```python
from build123d import *

# Parameters (mm, degrees)
TOP_BOW_EXTRUSION_DEPTH              = 56.86004
PORT_STARBOARD_CUT_DEPTH             = 38.529378828
PORT_STARBOARD_CUT_DEPTH_BACK        = 38.529527124
FORE_AFT_BOW_WRAPUP_EXTRUSTION_REACH = 76.36
SCALE_2_SCALE                        = 2
SHELL2_T                             = 2.54


with BuildPart() as part:
    # Cross-Section C Sketch → Fore-Aft Loft section 0
    with BuildSketch(Plane.XY.offset(76.2)):
        Polygon((-0.000593186, -30.406404979), (37.528192355, -12.906444879), (37.528192355, 26.453635249), (-37.529378728, 26.453635249), (-37.529378728, -12.906444879), align=None)
    # Cross-Section B Sketch → Fore-Aft Loft section 1
    with BuildSketch(Plane.XY):
        Polygon((-0.000593186, -30.406404979), (37.528192355, -12.906444879), (37.528192355, 26.453635249), (-37.529378728, 26.453635249), (-37.529378728, -12.906444879), align=None)
    # Cross-Section A Sketch → Fore-Aft Loft section 2
    with BuildSketch(Plane(origin=(0, 0, -76.2), x_dir=(-1, 0, 0), z_dir=(0, 0, -1))):
        Polygon((-0.000593186, -30.406404979), (37.528192355, -12.906444879), (37.528192355, 26.453635249), (-37.529378728, 26.453635249), (-37.529378728, -12.906444879), align=None)
    loft()

    # Top Bow Profile → Top Bow Extrusion (add)
    with BuildSketch(Plane(origin=(0, 26.453635249, 0), x_dir=(1, 0, 0), z_dir=(0, 1, 0))):
        Polygon((37.529378728, 76.2), (0, 150.560276873), (-37.528192355, 76.2), align=None)
    extrude(amount=-TOP_BOW_EXTRUSION_DEPTH)

    # Port-Starboard Profile → Port-Starboard Cut (cut, two sides)
    with BuildSketch(Plane(origin=(0, 0, 0), x_dir=(0, 0, -1), z_dir=(1, 0, 0))) as port_starboard_cut_sk:
        with BuildLine():
            ThreePointArc((76.2, -30.406404979), (122.925878209, -14.460087823), (150.560276873, 26.453635249))
            Line((150.560276873, 26.453635249), (150.560276873, -30.406404979))
            Line((150.560276873, -30.406404979), (76.2, -30.406404979))
        make_face()
    extrude(amount=PORT_STARBOARD_CUT_DEPTH, mode=Mode.SUBTRACT)
    extrude(port_starboard_cut_sk.sketch, amount=-PORT_STARBOARD_CUT_DEPTH_BACK, mode=Mode.SUBTRACT)

    # Fore-Aft Bow Construction Sketch → Fore-aft bow wrapup extrustion (cut, up to next)
    with BuildSketch(Plane.XY.offset(-76.2), mode=Mode.PRIVATE) as fore_aft_bow_wrapup_extrustion_sk1:
        Polygon((0.000593186, -30.406404979), (37.529378728, -30.406404979), (37.529378728, -12.906444879), align=None)
    fore_aft_bow_wrapup_extrustion_tool1 = extrude(fore_aft_bow_wrapup_extrustion_sk1.sketch, amount=-FORE_AFT_BOW_WRAPUP_EXTRUSTION_REACH, mode=Mode.PRIVATE) & part.part
    add(fore_aft_bow_wrapup_extrustion_tool1.solids().sort_by_distance((25.019784, -24.573085, -76.2))[0], mode=Mode.SUBTRACT)
    # Fore-Aft Bow Construction Sketch → Fore-aft bow wrapup extrustion (cut, up to next)
    with BuildSketch(Plane.XY.offset(-76.2), mode=Mode.PRIVATE) as fore_aft_bow_wrapup_extrustion_sk2:
        Polygon((-37.528192355, -30.406404979), (0.000593186, -30.406404979), (-37.528192355, -12.906444879), align=None)
    fore_aft_bow_wrapup_extrustion_tool2 = extrude(fore_aft_bow_wrapup_extrustion_sk2.sketch, amount=-FORE_AFT_BOW_WRAPUP_EXTRUSTION_REACH, mode=Mode.PRIVATE) & part.part
    add(fore_aft_bow_wrapup_extrustion_tool2.solids().sort_by_distance((-25.018597, -24.573085, -76.2))[0], mode=Mode.SUBTRACT)


with BuildPart() as part_1:
    # Scale 2: scaled about (-0.000240035, 2.235376986, -18.845056047)
    add(part.part.scale(SCALE_2_SCALE).moved(Location((0.000240035, -2.235376986, 18.845056047))))

    # Shell2 (no face opened: a closed hollow body)
    add(offset(amount=-SHELL2_T, mode=Mode.PRIVATE), mode=Mode.SUBTRACT)


solid = part_1.part
```
Source: CAD feature listing. Evaluate the final solid. Frame: model axes, mm. A direction names the side the tool comes from. Coordinates: 2 decimals unless noted, no trailing zeros. Write each loop counter-clockwise with the first axis right and the second up, starting at its lowest first coordinate (ties: lowest second). Pieces come first, ordered by that corner, then holes. Notation, with made-up numbers: (39, -16) -> (48, -16) arc R11 cw to (48, -7) -> close; hole circle Ø7 at (-9, 23.25). An arc over 180 degrees is marked (long way). Return JSON: item names as keys, results as strings. Group by question number.
1) Contact query for flat-ended pins moving along their axis: P1, Ø4, axis at x = -25, z = -32, coming from the -Y side; P2, Ø1.5, axis at y = 13, z = -226.5, coming from the -X side; P3, Ø2, axis at y = -38.5, z = -175, coming from the +X side. Output: stop coordinate, or through.
2) Set-up query: faces 1 (the face through (46.395, 14.147, -190.35)), 2 (the face through (36.613, -43.173, -160.317)). Return all of +Z, -Z, +X, -X, +Y, -Y with unobstructed straight access to the full face (end or side cutting, diameter ignored); none if empty.
3) Section query A-A, the plane z = -194. Return loops of the section in (x, y).
4) Mould query, pull axis X, two halves, no side actions, for faces 3 (the face through (-45.342, 14.147, -192.432)), 4 (the face through (-1, 48.132, -8)), 5 (the face through (-1, 50.672, -8)). Classes: +X half, -X half, draft (parallel to the pull), parting line (faces both ways), or undercut.
5) Ray query, line 1 along X through (y, z) = (2, -65.5); line 2 along Z through (x, y) = (28.5, -24.5); line 3 along Z through (x, y) = (-2, -44.5). Return the intervals inside material, ascending.
From the geometry:
{
 "1": {"P1": "y = -52.32", "P2": "x = -28.53", "P3": "x = 54.42"},
 "2": {"face 1": "-Z, +X, +Y, -Y", "face 2": "none"},
 "3": {"outline": "(-44.55, -42.27) -> (-26.99, -50.46) -> (26.99, -50.46) -> (44.55, -42.27) -> (44.55, 50.67) -> (-44.55, 50.67) -> close; hole (-41.71, -40.8) -> (-26.92, -47.69) -> (26.92, -47.69) -> (41.71, -40.8) -> (41.71, 48.13) -> (-41.71, 48.13) -> close"},
 "4": {"face 3": "-X half", "face 4": "undercut", "face 5": "draft"},
 "5": {"line 1": "-75.06 to -72.52, 72.52 to 75.06", "line 2": "-225.81 to -220.17, 168.71 to 171.25", "line 3": "-206.34 to -200.83, 168.71 to 171.25"}
}
